from build123d import *

# Parameters (mm, degrees)
SKETCH1_W           = 260.604
SKETCH1_H           = 49.1998
BOSS_EXTRUDE1_DEPTH = 4.7625
SKETCH2_R           = 4.7625
BOSS_EXTRUDE2_DEPTH = 9.525
SKETCH3_W           = 4.7752
SKETCH3_H           = 4.7752
BOSS_EXTRUDE3_DEPTH = 6.35
SKETCH4_W           = 260.604
SKETCH4_H           = 6.35
CUT_EXTRUDE1_DEPTH  = 4.7625
SKETCH5_W           = 260.604
SKETCH5_H           = 6.35
CUT_EXTRUDE2_DEPTH  = 4.7625
FILLET1_R           = 1.27


with BuildPart() as part:
    # Sketch1 → Boss-Extrude1 (new, symmetric)
    with BuildSketch(Plane.XY):
        Rectangle(SKETCH1_W, SKETCH1_H)
    extrude(amount=BOSS_EXTRUDE1_DEPTH, both=True)

    # Sketch2 → Boss-Extrude2 (add)
    with BuildSketch(Plane(origin=(130.302, 0, 0), x_dir=(0, 0, -1), z_dir=(1, 0, 0))):
        Circle(SKETCH2_R)
    boss_extrude2 = extrude(amount=BOSS_EXTRUDE2_DEPTH)

    # Sketch3 → Boss-Extrude3 (add)
    with BuildSketch(Plane(origin=(139.827, 0, 0), x_dir=(0, 0, -1), z_dir=(1, 0, 0))):
        Rectangle(SKETCH3_W, SKETCH3_H)
    boss_extrude3 = extrude(amount=BOSS_EXTRUDE3_DEPTH)

    # Mirror1: Boss-Extrude2, Boss-Extrude3 across plane
    add(boss_extrude2.mirror(Plane(origin=(0, 0, 0), x_dir=(0, 0, 1), z_dir=(1, 0, 0))))
    add(boss_extrude3.mirror(Plane(origin=(0, 0, 0), x_dir=(0, 0, 1), z_dir=(1, 0, 0))))

    # Sketch4 → Cut-Extrude1 (cut)
    with BuildSketch(Plane.XY.offset(4.7625)):
        with Locations((0, 21.4249)):
            Rectangle(SKETCH4_W, SKETCH4_H)
    extrude(amount=-CUT_EXTRUDE1_DEPTH, mode=Mode.SUBTRACT)

    # Sketch5 → Cut-Extrude2 (cut)
    with BuildSketch(Plane(origin=(0, 0, -4.7625), x_dir=(-1, 0, 0), z_dir=(0, 0, -1))):
        with Locations((0, -21.4249)):
            Rectangle(SKETCH5_W, SKETCH5_H)
    extrude(amount=-CUT_EXTRUDE2_DEPTH, mode=Mode.SUBTRACT)

    # Fillet1
    fillet1_edges = [part.edges().sort_by_distance(p)[0] for p in [
        (0, 24.5999, 0),
        (0, -24.5999, 0),
    ]]
    fillet(fillet1_edges, radius=FILLET1_R)


solid = part.part
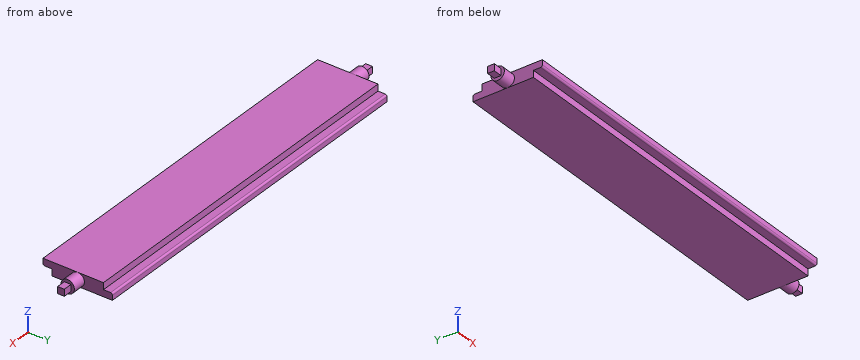
Can you work these out from the model? Positions are in its coordinate system, mm. Round coordinates to 2 decimals unless told otherwise and drop trailing zeros. Write each loop counter-clockwise with the first axis right and the second up, starting at its lowest first coordinate (ties: lowest second). Pieces come first, ordered by that corner, then holes. Notation, with made-up numbers: M 50.5,-18.5 L 73.5,-18.5 A27 ccw 73.5,19.5 Z; hole C 11.5,72.25 d10. An arc over 180 degrees is marked long. Use CSV: the item, a comma, the result in double quotes.
(1) I'm going to push flat-ended pins straight in: pin 1 (1.4 mm diameter, centred on x = 143.5, z = -0.5, fed in from +Y); pin 2 (4 mm diameter, centred on x = -143, y = -1, fed in from +Z); pin 3 (4 mm diameter, centred on x = 143, z = 1, fed in from -Y); pin 4 (5 mm diameter, centred on y = 3, z = -3, fed in from +X). Where does each tip first touch, or does it pass through?
Check values:
pin 1,"y = 2.39"
pin 2,"z = 2.39"
pin 3,"y = -2.39"
pin 4,"x = 146.18"
(2) Imagine slicing it at A-A (x = -25). Write out the boundary of the cut face in (y, z), plus the area to 3 significant figures.
Check values:
outline,"M -24.6,1.27 A1.27 ccw -23.33,0 L -18.25,0 L -18.25,-4.76 L 24.6,-4.76 L 24.6,-1.27 A1.27 ccw 23.33,0 L 18.25,0 L 18.25,4.76 L -24.6,4.76 Z"
area,"407 mm^2"
(3) I need wall thicknesses on line 1 along X through (y, z) = (10.5, 1.5); line 2 along X through (y, z) = (-2, -3); line 3 along Z through (x, y) = (-73, -20). Which ranges of each line are inside material? Lowest first, please.
Check values:
line 1,"-130.3 to 130.3"
line 2,"-139.83 to 139.83"
line 3,"0 to 4.76"
(4) Imagine slicing it at B-B (y = 9). Write out the boundary of the cut face in (x, z).
Check values:
outline,"M -130.3,-4.76 L 130.3,-4.76 L 130.3,4.76 L -130.3,4.76 Z"
